Here's how the part is built. I have some questions about the finished solid (model axes, mm). Coordinates: 2 decimals unless noted, no trailing zeros. Order: outer loops, then holes, each group sorted by start corner. A loop starts at its lowest first (then second) coordinate and runs counter-clockwise, first axis right, second up. Notation, with made-up numbers: (70, 66.25) - (83, 66.25) arc R31 ccw to (83, 92.25) - close; hole circle Ø7 at (30, -9.75). An arc over 180 degrees is marked (long way). Answer in a Markdown table with one row per item. Add a question column.
Item 1: I want a section at D-D (x = 19.5). Please give me the cut outline in (y, z).
Item 2: Will these pins go through, and if not, where does the flat tip stop? pin 1 Ø0.9 at (y, z) = (1.5, -27) entering from -X; pin 2 Ø0.9 at (y, z) = (1.5, 24.5) entering from +X; pin 3 Ø1 at (y, z) = (0.5, -1) entering from +X.
Item 3: If I drill on line 1 along Z through (x, y) = (0, 2.8); line 2 along X through (y, z) = (1.6, 8.5); line 3 along Z through (x, y) = (-15.7, 1.1), over which ranges is the centre line in solid material (lowest first)? Write a range as from..to.
Item 4: I want a section at A-A (x = 36.5). Please give me the cut outline in (y, z), plus the area to 3 significant figures.
Item 5: I want a section at C-C (x = 9). Please give me the cut outline in (y, z), plus the area to 3 significant figures.
Item 6: I want a section at B-B (y = 1.9). Count the separate pieces of the cut face and the enclosed holes in it, plus the area to 3 significant figures.
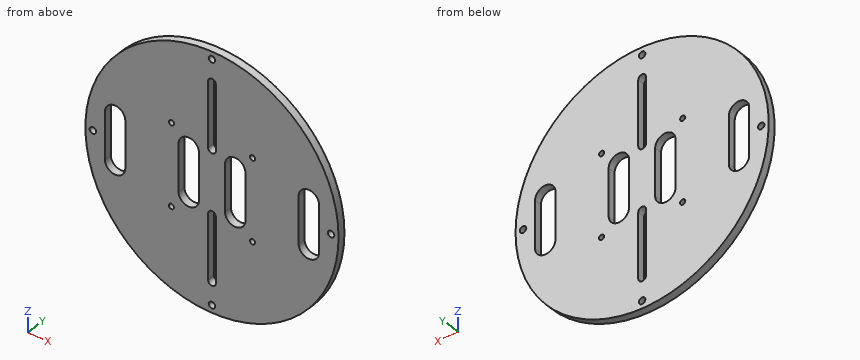
```python
from build123d import *

# Parameters (mm, degrees)
SKETCH_1_R                      = 49
EXTRUDE_1_DEPTH                 = 3
CUT_EXTRUDE_1_DEPTH             = 4
PATTERN_CIRCULAR_2_COUNT        = 2
CUT_EXTRUDE_3_DEPTH             = 4
PATTERN_LINEAR_1_COUNT          = 2
PATTERN_LINEAR_1_PITCH          = 28.5
PATTERN_CIRCULAR_5_COUNT        = 2
PATTERN_CIRCULAR_5_COPY_1_DEPTH = 4
SKETCH_14_R                     = 1.25
CUT_EXTRUDE_4_DEPTH             = 4
PATTERN_CIRCULAR_6_COUNT        = 4
SKETCH_8_R                      = 1
CUT_EXTRUDE_5_DEPTH             = 4
PATTERN_CIRCULAR_7_COUNT        = 4


with BuildPart() as part:
    # 草图1 → 凸台-拉伸1 (new body)
    with BuildSketch(Plane(origin=(0, 0, 0), x_dir=(1, 0, 0), z_dir=(0, 1, 0))):
        Circle(SKETCH_1_R)
    extrude(amount=EXTRUDE_1_DEPTH)

    # 草图6 → 切除-拉伸1 (cut, through all)
    with BuildSketch(Plane(origin=(0, 3, 0), x_dir=(1, 0, 0), z_dir=(0, 1, 0))):
        with BuildLine():
            Line((-1.5, 12.3), (-1.5, 37.3))
            ThreePointArc((-1.5, 37.3), (0, 38.8), (1.5, 37.3))
            Line((1.5, 37.3), (1.5, 12.3))
            ThreePointArc((1.5, 12.3), (0, 10.8), (-1.5, 12.3))
        make_face()
    cut_extrude_1 = extrude(amount=-CUT_EXTRUDE_1_DEPTH, mode=Mode.SUBTRACT)

    # 阵列(圆周)2: 切除-拉伸1 ×2 about axis
    pattern_circular_2_axis = Axis((0, 0, 0), (0, 1, 0))
    for i in range(1, PATTERN_CIRCULAR_2_COUNT):
        add(cut_extrude_1.rotate(pattern_circular_2_axis, i * 360 / PATTERN_CIRCULAR_2_COUNT), mode=Mode.SUBTRACT)

    # 草图9 → 切除-拉伸3 (cut, through all)
    with BuildSketch(Plane(origin=(0, 3, 0), x_dir=(1, 0, 0), z_dir=(0, 1, 0))):
        with BuildLine():
            Line((-12.95, -9), (-12.95, 9))
            ThreePointArc((-12.95, 9), (-9, 12.95), (-5.05, 9))
            Line((-5.05, 9), (-5.05, -9))
            ThreePointArc((-5.05, -9), (-9, -12.95), (-12.95, -9))
        make_face()
    cut_extrude_3 = extrude(amount=-CUT_EXTRUDE_3_DEPTH, mode=Mode.SUBTRACT)

    # 阵列(线性)1: 切除-拉伸3 ×2
    with Locations(*[(-i * PATTERN_LINEAR_1_PITCH, 0, 0) for i in range(1, PATTERN_LINEAR_1_COUNT)]):
        add(cut_extrude_3, mode=Mode.SUBTRACT)

    # 阵列(圆周)5: 切除-拉伸3 ×2 about axis
    pattern_circular_5_axis = Axis((0, 0, 0), (0, 1, 0))
    for i in range(1, PATTERN_CIRCULAR_5_COUNT):
        add(cut_extrude_3.rotate(pattern_circular_5_axis, i * 360 / PATTERN_CIRCULAR_5_COUNT), mode=Mode.SUBTRACT)

    # 阵列(圆周)5 copy 1 sketch → 阵列(圆周)5 copy 1 (cut, through all)
    with BuildSketch(Plane(origin=(28.5, 3, 0), x_dir=(-1, 0, 0), z_dir=(0, 1, 0))):
        with BuildLine():
            Line((-12.95, -9), (-12.95, 9))
            ThreePointArc((-12.95, 9), (-9, 12.95), (-5.05, 9))
            Line((-5.05, 9), (-5.05, -9))
            ThreePointArc((-5.05, -9), (-9, -12.95), (-12.95, -9))
        make_face()
    extrude(amount=-PATTERN_CIRCULAR_5_COPY_1_DEPTH, mode=Mode.SUBTRACT)

    # 草图14 → 切除-拉伸4 (cut, through all)
    with BuildSketch(Plane(origin=(0, 3, 0), x_dir=(1, 0, 0), z_dir=(0, 1, 0))):
        with Locations((0, 46.1)):
            Circle(SKETCH_14_R)
    cut_extrude_4 = extrude(amount=-CUT_EXTRUDE_4_DEPTH, mode=Mode.SUBTRACT)

    # 阵列(圆周)6: 切除-拉伸4 ×4 about axis
    pattern_circular_6_axis = Axis((0, 0, 0), (0, 1, 0))
    for i in range(1, PATTERN_CIRCULAR_6_COUNT):
        add(cut_extrude_4.rotate(pattern_circular_6_axis, i * 360 / PATTERN_CIRCULAR_6_COUNT), mode=Mode.SUBTRACT)

    # 草图8 → 切除-拉伸5 (cut, through all)
    with BuildSketch(Plane(origin=(0, 3, 0), x_dir=(1, 0, 0), z_dir=(0, 1, 0))):
        with Locations((-15.7, 15.7)):
            Circle(SKETCH_8_R)
    cut_extrude_5 = extrude(amount=-CUT_EXTRUDE_5_DEPTH, mode=Mode.SUBTRACT)

    # 阵列(圆周)7: 切除-拉伸5 ×4 about axis
    pattern_circular_7_axis = Axis((0, 0, 0), (0, 1, 0))
    for i in range(1, PATTERN_CIRCULAR_7_COUNT):
        add(cut_extrude_5.rotate(pattern_circular_7_axis, i * 360 / PATTERN_CIRCULAR_7_COUNT), mode=Mode.SUBTRACT)


solid = part.part
```
Values follow:
| question | item | result |
|---|---|---|
| 1 | outline | (0, -44.95) - (3, -44.95) - (3, 44.95) - (0, 44.95) - close |
| 2 | pin 1 | stops at x = -41.18 |
| 2 | pin 2 | stops at x = 42.69 |
| 2 | pin 3 | stops at x = 49 |
| 3 | line 1 | z = -49..-47.35, -44.85..-38.8, -10.8..10.8, 38.8..44.85, 47.35..49 |
| 3 | line 2 | x = -48.26..-41.45, -33.55..-12.95, -5.05..5.05, 12.95..33.55, 41.45..48.26 |
| 3 | line 3 | z = -46.42..-16.7, -14.7..14.7, 16.7..46.42 |
| 4 | outline | (0, -32.69) - (3, -32.69) - (3, -12.82) - (0, -12.82) - close; (0, 12.82) - (3, 12.82) - (3, 32.69) - (0, 32.69) - close |
| 4 | area | 119 mm^2 |
| 5 | outline | (0, -48.17) - (3, -48.17) - (3, -12.95) - (0, -12.95) - close; (0, 12.95) - (3, 12.95) - (3, 48.17) - (0, 48.17) - close |
| 5 | area | 211 mm^2 |
| 6 | separate pieces | 1 |
| 6 | enclosed holes | 14 |
| 6 | area | 6,580 mm^2 |
